Source: three-view drawing plus pictorial views. Frame: mm from the lowest corner of the part. Coordinates: 2 decimals unless noted, no trailing zeros. Loops run counter-clockwise (first coordinate to the right, second up) from the corner with the lowest first, then second, coordinate; pieces in that order, holes last. Notation, with made-up numbers: (89, 73.25) - (110, 73.25) arc R20 ccw to (110, 79.25) - close; hole circle Ø10 at (51, 68.25). An arc over 180 degrees is marked (long way). Return JSON: item names as keys, results as strings.
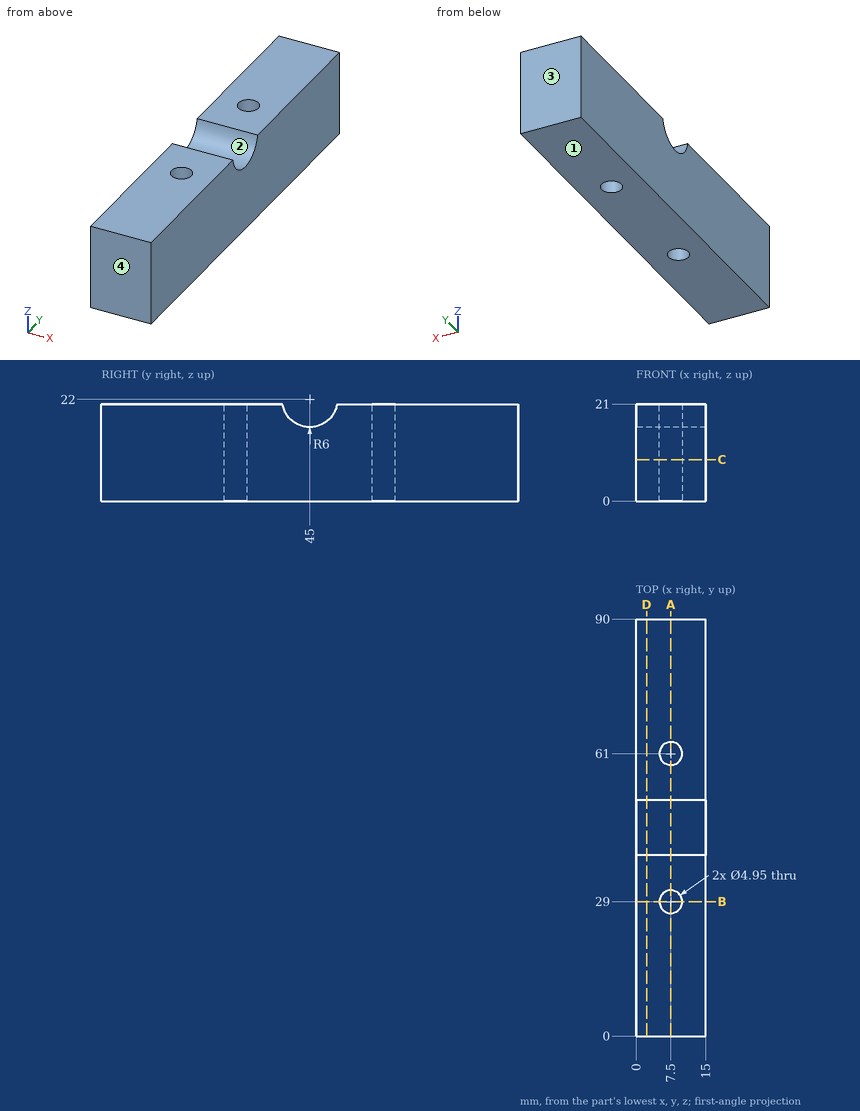
Item 1: Mould query, pull axis Y, two halves, no side actions, for the marked faces 1, 2, 3 and 4. Classes: +Y half, -Y half, draft (parallel to the pull), parting line (faces both ways), or undercut.
Worked out:
{"face 1": "draft", "face 2": "undercut", "face 3": "+Y half", "face 4": "-Y half"}
Item 2: First-contact query: pin 1 Ø4.5 at (x, y) = (7.5, 29) entering from -Z; pin 2 Ø1 at (x, z) = (13, 15) entering from -Y. Flat tips, straight axial feed; report the tip coordinate or a pass-through.
Worked out:
{"pin 1": "through", "pin 2": "y = 0"}
Item 3: Section query C-C, the plane z = 9. Return loops of the section in (x, y) (3 decimals), and give its area (3 significant figures).
Worked out:
{"outline": "(0, 0) - (15, 0) - (15, 90) - (0, 90) - close; hole circle Ø4.95 at (7.5, 29); hole circle Ø4.95 at (7.5, 61)", "area": "1,310 mm^2"}
Item 4: Section query D-D, the plane x = 2.25. Return loops of the section in (y, z), and give its area (3 significant figures).
Worked out:
{"outline": "(0, 0) - (90, 0) - (90, 21) - (50.92, 21) arc R6 cw to (39.08, 21) - (0, 21) - close", "area": "1,850 mm^2"}
Item 5: Ray query, probe 1 along Y at (x, z) = (7.5, 12.25) (3 decimals); probe 2 along Y at (x, z) = (5.5, 1); probe 3 along X at (y, z) = (61.5, 11.5). Return the intervals inside material, ascending. Write a range as from..to.
Worked out:
{"probe 1": "0..26.525, 31.475..58.525, 63.475..90", "probe 2": "0..27.54, 30.46..59.54, 62.46..90", "probe 3": "0..5.08, 9.92..15"}
Item 6: Section query B-B, the plane y = 29. Return loops of the section in (x, z) (3 decimals).
Worked out:
{"outline": "(0, 0) - (5.025, 0) - (5.025, 21) - (0, 21) - close; (9.975, 0) - (15, 0) - (15, 21) - (9.975, 21) - close"}
Item 7: Section query A-A, the plane x = 7.5. Return loops of the section in (y, z) (3 decimals), and give its area (3 significant figures).
Worked out:
{"outline": "(0, 0) - (26.525, 0) - (26.525, 21) - (0, 21) - close; (31.475, 0) - (58.525, 0) - (58.525, 21) - (50.916, 21) arc R6 cw to (39.084, 21) - (31.475, 21) - close; (63.475, 0) - (90, 0) - (90, 21) - (63.475, 21) - close", "area": "1,640 mm^2"}
